Check sheet for the modelled part. Datum: model origin and axes. Units: mm. A direction names the side the tool comes from. Round coordinates to 2 decimals unless told otherwise and drop trailing zeros. Write each loop counter-clockwise with the first axis right and the second up, starting at its lowest first coordinate (ties: lowest second). Pieces come first, ordered by that corner, then holes. Notation, with made-up numbers: (86, 30) - (139, 30) arc R29 ccw to (139, 60) - close; hole circle Ø9 at (68, 32). An arc over 180 degrees is marked (long way). Answer as a JSON object with one key per item and string values. Group by question number.
Item 1: Thickness scan on line 1 (Z direction, x = -4.25, y = -50); line 2 (X direction, y = -24.5, z = -0.75); line 3 (Y direction, x = -7.5, z = 4.5). Record the ranges inside material, lowest first.
Item 2: Sectioned sample at A-A on x = 0. Record the boundary of the cut face in (y, z), plus the area to 3 significant figures.
Item 3: Sectioned sample at B-B on z = 0. Record the boundary of the cut face in (x, y).
Item 4: Gauge pin test, flat ends, axial feed: P1, Ø9, axis at y = -41.5, z = -0.5, coming from the +X side; P2, Ø4, axis at x = 8, y = -3.5, coming from the +Z side; P3, Ø6, axis at x = 5.5, y = -6, coming from the -Z side. Record the tip position at first contact, or that the pin passes through.
Item 5: Set-up check for faces 1 (the flat face through (0, 0, 6)), 2 (the flat face through (0, -32, -4)), 3 (the flat face through (-9.165, -32, 0)): record each of +Z, -Z, +X, -X, +Y, -Y from which the full face is reachable in a straight line by a thin tool's end or side.
Item 6: Sectioned sample at C-C on y = -42. Record the boundary of the cut face in (x, z).
Item 7: Sectioned sample at D-D on z = 9. Record the boundary of the cut face in (x, y).
Autodesk Inventor part; units mm, degrees
ref_plane "YZ Plane" through (0, 0, 0) normal (1, 0, 0) x (0, 1, 0)
ref_plane "XZ Plane" through (0, 0, 0) normal (0, 1, 0) x (-1, 0, 0)
ref_plane "XY Plane" through (0, 0, 0) normal (0, 0, 1) x (1, 0, 0)
sketch "Sketch1" plane through (0, 0, 0) normal (0, 1, 0) x (-1, 0, 0)
  circle A0 centre (0, 0) radius 10
  dimension "d0" = 20
extrude "Extrusion1" add sketch "Sketch1" along normal blind 5
sketch "Sketch2" plane through (0, 0, 0) normal (0, -1, 0) x (1, 0, 0)
  line L0 (9.1652, 4) -> (-9.1652, 4)
  line L1 (-9.1652, 4) -> (-9.1652, -4)
  line L2 (-9.1652, -4) -> (9.1652, -4)
  line L3 (9.1652, -4) -> (9.1652, 4)
  circle A0 centre (0, 0) radius 10
  circle A1 centre (0, 0) radius 10
  dimension "d3" = 8
extrude "Extrusion2" add sketch "Sketch2" along normal blind 65 contours L3 L2 L1 L0
properties part number "rack"
Completed:
{
 "1": {"line 1": "-4 to 4", "line 2": "-9.17 to 9.17", "line 3": "0 to 5"},
 "2": {"outline": "(-65, -4) - (0, -4) - (0, -10) - (5, -10) - (5, 10) - (0, 10) - (0, 4) - (-65, 4) - close", "area": "620 mm²"},
 "3": {"outline": "(-10, 0) - (-9.17, 0) - (-9.17, -65) - (9.17, -65) - (9.17, 0) - (10, 0) - (10, 5) - (-10, 5) - close"},
 "4": {"P1": "x = 9.17", "P2": "z = 4", "P3": "z = -4"},
 "5": {"face 1": "+Z, +X, -X, -Y", "face 2": "-Z, +X, -X, -Y", "face 3": "+Z, -Z, -X, -Y"},
 "6": {"outline": "(-9.17, -4) - (9.17, -4) - (9.17, 4) - (-9.17, 4) - close"},
 "7": {"outline": "(-4.36, 0) - (4.36, 0) - (4.36, 5) - (-4.36, 5) - close"}
}
